from build123d import *

# Parameters (mm, degrees)
SKETCH_1_R            = 2.75
EXTRUDE_248_DEPTH     = 3
CUT_EXTRUDE_378_DEPTH = 1.3
SKETCH_3_R            = 1.5
EXTRUDE_479_DEPTH     = 28


with BuildPart() as part:
    # 草图1 → Extrude 248 (new body)
    with BuildSketch(Plane(origin=(0, 0, 0), x_dir=(1, 0, 0), z_dir=(0, 1, 0))):
        Circle(SKETCH_1_R)
    extrude(amount=EXTRUDE_248_DEPTH)

    # 草图2 → Cut-Extrude 378 (cut)
    with BuildSketch(Plane(origin=(0, 3, 0), x_dir=(1, 0, 0), z_dir=(0, 1, 0))):
        Polygon((1.443375673, 0), (0.721687836, 1.25), (-0.721687836, 1.25), (-1.443375673, 0), (-0.721687836, -1.25), (0.721687836, -1.25), align=None)
    extrude(amount=-CUT_EXTRUDE_378_DEPTH, mode=Mode.SUBTRACT)

    # 草图3 → Extrude 479 (add)
    with BuildSketch(Plane.XZ):
        Circle(SKETCH_3_R)
    extrude(amount=EXTRUDE_479_DEPTH)


solid = part.part
Part model, mm, in its own coordinate system. A direction names the side the tool comes from. Coordinates: 2 decimals unless noted, no trailing zeros. Write each loop counter-clockwise with the first axis right and the second up, starting at its lowest first coordinate (ties: lowest second). Pieces come first, ordered by that corner, then holes. Notation, with made-up numbers: (21, -23.75) - (76, -23.75) arc R21 ccw to (76, -10.75) - close; hole circle Ø5 at (78, 61). An arc over 180 degrees is marked (long way). Put each result on its own line as item: value.
1. Band-saw the part on A-A (x = 0). Write the cut outline in (y, z), then the cut area to 4 significant figures.
Final values:
outline: (-28, -1.5) - (0, -1.5) - (0, -2.75) - (3, -2.75) - (3, -1.25) - (1.7, -1.25) - (1.7, 1.25) - (3, 1.25) - (3, 2.75) - (0, 2.75) - (0, 1.5) - (-28, 1.5) - close
area: 97.25 mm²
2. Band-saw the part on C-C (y = -16). Write the cut outline in (x, z).
Final values:
outline: circle Ø3 at (0, 0)
3. Band-saw the part on B-B (z = 0.7). Write the cut outline in (x, y).
Final values:
outline: (-2.66, 0) - (-1.33, 0) - (-1.33, -28) - (1.33, -28) - (1.33, 0) - (2.66, 0) - (2.66, 3) - (1.04, 3) - (1.04, 1.7) - (-1.04, 1.7) - (-1.04, 3) - (-2.66, 3) - close
4. Flat gauge pins, fed straight in: pin 1 Ø2 at (x, z) = (0.5, 0) entering from +Y; pin 2 Ø2 at (y, z) = (-19.5, -0.5) entering from +X; pin 3 Ø1.5 at (y, z) = (-2.5, -2) entering from +X. Where does each tip first touch, or does it go through?
Final values:
pin 1: stops at y = 3
pin 2: stops at x = 1.5
pin 3: stops at x = 0.83
5. Band-saw the part on D-D (z = 2.1). Write the cut outline in (x, y).
Final values:
outline: (-1.78, 0) - (1.78, 0) - (1.78, 3) - (-1.78, 3) - close
6. Probe line 1 along Y through (x, z) = (-1.65, -2); line 2 along Y through (x, z) = (-0.9, 0.6); line 3 along Z through (x, y) = (0.1, -4). List the from-to ranges inside material, lowest first. Write a range as [from, to].
Final values:
line 1: y = [0, 3]
line 2: y = [-28, 1.7]
line 3: z = [-1.5, 1.5]
7. 3-axis set-ups, long thin cutter, end or side, ignore diameter. For faces 4 (the flat face through (1.088, 2.359, -0.616)), 5 (the flat face through (1.2, 0, 1.2)), 6 (the flat face through (0, -28, 0)): which of +Z, -Z, +X, -X, +Y, -Y reach the whole face in a straight line?
Final values:
face 4: +Y
face 5: -Y
face 6: +Z, -Z, +X, -X, -Y
8. Two-plate mould, pull along X, no slides. Class faces 1 (the flat face through (-1.3, 3, 0.6)), 2 (the cylindrical face through (-0.596, 1.479, 2.685)), 3 (the flat face through (0, 1.7, 0)): +X half, -X half, draft (parallel to the pull), parting line (faces both ways), or undercut.
Final values:
face 1: draft
face 2: parting line
face 3: undercut
